Check sheet for the modelled part. Datum: model origin and axes. Units: mm. Give positions to 0.01 mm unless a question says otherwise; leave off trailing zeros. Loops run counter-clockwise (first coordinate to the right, second up) from the corner with the lowest first, then second, coordinate; pieces in that order, holes last. Notation, with made-up numbers: (21.25, -23.5) - (34.25, -23.5) arc R23 ccw to (34.25, 7.5) - close; hole circle Ø10 at (-10, 29.25). An arc over 180 degrees is marked (long way). Use one line per item in the form item = value.
from build123d import *

# Parameters (mm, degrees)
F1_DEPTH = 3.175


with BuildPart() as f1:
    # F0 (on Top) → F1 (new body)
    with BuildSketch(Plane.XY):
        with BuildLine():
            Line((-50.8, 0), (-47.625, 0))
            ThreePointArc((-47.625, 0), (-35.8063708312, 31.4013444441), (-6.2163099045, 47.2175615229))
            Line((-6.2163099045, 47.2175615229), (-6.6307305648, 50.3653989578))
            ThreePointArc((-6.6307305648, 50.3653989578), (-38.1934622199, 33.4947674071), (-50.8, 0))
        make_face()
        with BuildLine():
            ThreePointArc((-47.2175615229, -6.2163099045), (-47.5230312192, -3.1148240296), (-47.625, 0))
            Line((-47.625, 0), (-50.8, 0))
            ThreePointArc((-50.8, 0), (-50.6912333005, -3.3224789649), (-50.3653989578, -6.6307305648))
            Line((-50.3653989578, -6.6307305648), (-47.2175615229, -6.2163099045))
        make_face()
        with BuildLine():
            Line((0, -50.8), (0, -47.625))
            ThreePointArc((0, -47.625), (-31.4013444441, -35.8063708312), (-47.2175615229, -6.2163099045))
            Line((-47.2175615229, -6.2163099045), (-50.3653989578, -6.6307305648))
            ThreePointArc((-50.3653989578, -6.6307305648), (-33.4947674071, -38.1934622199), (0, -50.8))
        make_face()
        with BuildLine():
            Line((50.8, 0), (47.625, 0))
            ThreePointArc((47.625, 0), (35.8063708312, -31.4013444441), (6.2163099045, -47.2175615229))
            Line((6.2163099045, -47.2175615229), (6.6307305648, -50.3653989578))
            ThreePointArc((6.6307305648, -50.3653989578), (38.1934622199, -33.4947674071), (50.8, 0))
        make_face()
        with BuildLine():
            ThreePointArc((0, 47.625), (31.4013444441, 35.8063708312), (47.2175615229, 6.2163099045))
            Line((47.2175615229, 6.2163099045), (50.3653989578, 6.6307305648))
            ThreePointArc((50.3653989578, 6.6307305648), (33.4947674071, 38.1934622199), (0, 50.8))
            Line((0, 50.8), (0, 47.625))
        make_face()
        with BuildLine():
            ThreePointArc((-6.2163099045, 47.2175615229), (-3.1148240296, 47.5230312192), (0, 47.625))
            Line((0, 47.625), (0, 50.8))
            ThreePointArc((0, 50.8), (-3.3224789649, 50.6912333005), (-6.6307305648, 50.3653989578))
            Line((-6.6307305648, 50.3653989578), (-6.2163099045, 47.2175615229))
        make_face()
        with BuildLine():
            ThreePointArc((47.2175615229, 6.2163099045), (47.5230312192, 3.1148240296), (47.625, 0))
            Line((47.625, 0), (50.8, 0))
            ThreePointArc((50.8, 0), (50.6912333005, 3.3224789649), (50.3653989578, 6.6307305648))
            Line((50.3653989578, 6.6307305648), (47.2175615229, 6.2163099045))
        make_face()
        with BuildLine():
            Line((6.6307305648, -50.3653989578), (6.2163099045, -47.2175615229))
            ThreePointArc((6.2163099045, -47.2175615229), (3.1148240296, -47.5230312192), (0, -47.625))
            Line((0, -47.625), (0, -50.8))
            ThreePointArc((0, -50.8), (3.3224789649, -50.6912333005), (6.6307305648, -50.3653989578))
        make_face()
        with BuildLine():
            Line((-3.175, 0), (-1.5875, 0))
            ThreePointArc((-1.5875, 0), (-1.1935456944, 1.0467114815), (-0.2072103301, 1.5739187174))
            Line((-0.2072103301, 1.5739187174), (-0.4144206603, 3.1478374349))
            ThreePointArc((-0.4144206603, 3.1478374349), (-2.3870913887, 2.0934229629), (-3.175, 0))
        make_face()
        with BuildLine():
            ThreePointArc((-1.5739187174, -0.2072103301), (-1.5841010406, -0.1038274677), (-1.5875, 0))
            Line((-1.5875, 0), (-3.175, 0))
            ThreePointArc((-3.175, 0), (-3.1682020813, -0.2076549353), (-3.1478374349, -0.4144206603))
            Line((-3.1478374349, -0.4144206603), (-1.5739187174, -0.2072103301))
        make_face()
        with BuildLine():
            Line((0, -3.175), (0, -1.5875))
            ThreePointArc((0, -1.5875), (-1.0467114815, -1.1935456944), (-1.5739187174, -0.2072103301))
            Line((-1.5739187174, -0.2072103301), (-3.1478374349, -0.4144206603))
            ThreePointArc((-3.1478374349, -0.4144206603), (-2.0934229629, -2.3870913887), (0, -3.175))
        make_face()
        with BuildLine():
            Line((0.4144206603, -3.1478374349), (0.2072103301, -1.5739187174))
            ThreePointArc((0.2072103301, -1.5739187174), (0.1038274677, -1.5841010406), (0, -1.5875))
            Line((0, -1.5875), (0, -3.175))
            ThreePointArc((0, -3.175), (0.2076549353, -3.1682020813), (0.4144206603, -3.1478374349))
        make_face()
        with BuildLine():
            Line((3.175, 0), (1.5875, 0))
            ThreePointArc((1.5875, 0), (1.1935456944, -1.0467114815), (0.2072103301, -1.5739187174))
            Line((0.2072103301, -1.5739187174), (0.4144206603, -3.1478374349))
            ThreePointArc((0.4144206603, -3.1478374349), (2.3870913887, -2.0934229629), (3.175, 0))
        make_face()
        with BuildLine():
            ThreePointArc((1.5739187174, 0.2072103301), (1.5841010406, 0.1038274677), (1.5875, 0))
            Line((1.5875, 0), (3.175, 0))
            ThreePointArc((3.175, 0), (3.1682020813, 0.2076549353), (3.1478374349, 0.4144206603))
            Line((3.1478374349, 0.4144206603), (1.5739187174, 0.2072103301))
        make_face()
        with BuildLine():
            ThreePointArc((0, 1.5875), (1.0467114815, 1.1935456944), (1.5739187174, 0.2072103301))
            Line((1.5739187174, 0.2072103301), (3.1478374349, 0.4144206603))
            ThreePointArc((3.1478374349, 0.4144206603), (2.0934229629, 2.3870913887), (0, 3.175))
            Line((0, 3.175), (0, 1.5875))
        make_face()
        with BuildLine():
            ThreePointArc((-0.2072103301, 1.5739187174), (-0.1038274677, 1.5841010406), (0, 1.5875))
            Line((0, 1.5875), (0, 3.175))
            ThreePointArc((0, 3.175), (-0.2076549353, 3.1682020813), (-0.4144206603, 3.1478374349))
            Line((-0.4144206603, 3.1478374349), (-0.2072103301, 1.5739187174))
        make_face()
        with BuildLine():
            ThreePointArc((-0.4144206603, 3.1478374349), (-0.2076549353, 3.1682020813), (0, 3.175))
            Line((0, 3.175), (0, 47.625))
            ThreePointArc((0, 47.625), (-3.1148240296, 47.5230312192), (-6.2163099045, 47.2175615229))
            Line((-6.2163099045, 47.2175615229), (-0.4144206603, 3.1478374349))
        make_face()
        with BuildLine():
            ThreePointArc((-3.1478374349, -0.4144206603), (-3.1682020813, -0.2076549353), (-3.175, 0))
            Line((-3.175, 0), (-47.625, 0))
            ThreePointArc((-47.625, 0), (-47.5230312192, -3.1148240296), (-47.2175615229, -6.2163099045))
            Line((-47.2175615229, -6.2163099045), (-3.1478374349, -0.4144206603))
        make_face()
        with BuildLine():
            Line((6.2163099045, -47.2175615229), (0.4144206603, -3.1478374349))
            ThreePointArc((0.4144206603, -3.1478374349), (0.2076549353, -3.1682020813), (0, -3.175))
            Line((0, -3.175), (0, -47.625))
            ThreePointArc((0, -47.625), (3.1148240296, -47.5230312192), (6.2163099045, -47.2175615229))
        make_face()
        with BuildLine():
            ThreePointArc((3.1478374349, 0.4144206603), (3.1682020813, 0.2076549353), (3.175, 0))
            Line((3.175, 0), (47.625, 0))
            ThreePointArc((47.625, 0), (47.5230312192, 3.1148240296), (47.2175615229, 6.2163099045))
            Line((47.2175615229, 6.2163099045), (3.1478374349, 0.4144206603))
        make_face()
    extrude(amount=F1_DEPTH)


solid = f1.part
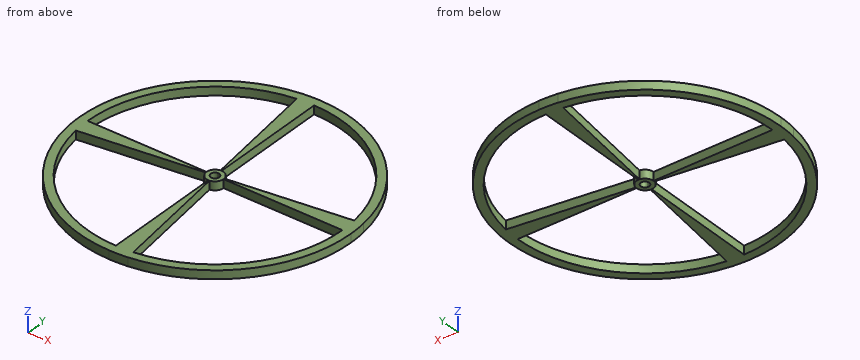
Item 1: Gauge pin test, flat ends, axial feed: P1, Ø1.5, axis at y = 10, z = 2, coming from the -X side; P2, Ø3, axis at x = -13.5, y = 3, coming from the +Z side; P3, Ø1, axis at y = -18.5, z = 1.5, coming from the -X side; P4, Ø1.6, axis at x = -17, z = 2, coming from the +Y side. Record the tip position at first contact, or that the pin passes through.
Answer block:
P1 = -49.95
P2 = through
P3 = -47.5
P4 = 48.15
Item 2: Section check B-B on x = -22.5. Record the boundary of the cut face in (y, z) (3 decimals).
Answer block:
outline = (-45.545, 0) - (-41.975, 0) - (-41.975, 3.175) - (-45.545, 3.175) - close; (-2.962, 0) - (0, 0) - (0, 3.175) - (-2.962, 3.175) - close; (41.975, 0) - (45.545, 0) - (45.545, 3.175) - (41.975, 3.175) - close
Item 3: Section check A-A on y = 35. Record the boundary of the cut face in (x, z) (3 decimals).
Answer block:
outline = (-36.819, 0) - (-32.298, 0) - (-32.298, 3.175) - (-36.819, 3.175) - close; (-4.608, 0) - (0, 0) - (0, 3.175) - (-4.608, 3.175) - close; (32.298, 0) - (36.819, 0) - (36.819, 3.175) - (32.298, 3.175) - close
Item 4: Section check C-C on z = 0.8. Give the number of separate pieces and of enclosed holes in the cut face, then the cut area to 3 significant figures.
Answer block:
separate_pieces = 1
enclosed_holes = 5
area = 1,600 mm2
Item 5: Thickness scan on L1, parallel to Y at x = 39, z = 1.4; L2, parallel to Y at x = -11, z = 1.1; L3, parallel to X at y = -18, z = 0.3. Record the ranges inside material, lowest first.
Answer block:
L1 = -32.55 to -27.33, 0 to 5.13, 27.33 to 32.55
L2 = -49.59 to -46.34, -1.45 to 0, 46.34 to 49.59
L3 = -47.5 to -44.09, 0 to 2.37, 44.09 to 47.5
